Could you check a few things on this model? Use its own coordinates, in mm. A direction names the side the tool comes from. Give positions to 0.01 mm unless a question says otherwise; leave off trailing zeros. Loops run counter-clockwise (first coordinate to the right, second up) from the corner with the lowest first, then second, coordinate; pieces in that order, holes last. Notation, with made-up numbers: (44.5, 33) - (89.5, 33) arc R32 ccw to (89.5, 72) - close; hole circle Ø9 at (36, 44). An arc over 180 degrees is marked (long way). Use CSV: the item, a comma, the result in double quotes.
from build123d import *

# Parameters (mm, degrees)
BOSS_EXTRUDE1_DEPTH      = 30
BOSS_EXTRUDE1_DEPTH_BACK = 30
BOSS_EXTRUDE2_DEPTH      = 3.2
SKETCH3_R                = 1.35
CUT_EXTRUDE1_DEPTH       = 86.695011246
SKETCH4_R                = 6.35
SKETCH4_R_2              = 1.35
BOSS_EXTRUDE3_DEPTH      = 6
CHAMFER1_SIZE            = 6
FILLET1_R                = 5
SKETCH5_W                = 2.4
SKETCH5_H                = 8
BOSS_EXTRUDE4_DEPTH      = 60
FILLET2_R                = 5
FILLET3_R                = 10


with BuildPart() as part:
    # Sketch1 → Boss-Extrude1 (new, two sides: drawn at the far end of the back side and taken through both)
    with BuildSketch(Plane(origin=(0, 0, 0), x_dir=(0, 0, -1), z_dir=(1, 0, 0)).offset(-BOSS_EXTRUDE1_DEPTH_BACK)):
        Polygon((-8, 54.174772512), (-46.414198462, 60.948232143), (-46.414198462, 57.901952308), (-1.6, 50), (-1.6, 0), (0, 0), (0, 50), align=None)
    extrude(amount=BOSS_EXTRUDE1_DEPTH + BOSS_EXTRUDE1_DEPTH_BACK)

    # Sketch2 → Boss-Extrude2 (add)
    with BuildSketch(Plane(origin=(30, 0, 0), x_dir=(0, 0, -1), z_dir=(1, 0, 0))):
        Polygon((0, 0), (0, 107.45890736), (-46.414198462, 107.45890736), (-46.414198462, 57.901952308), (-1.6, 0), align=None)
    boss_extrude2 = extrude(amount=BOSS_EXTRUDE2_DEPTH)

    # Mirror1: Boss-Extrude2 across plane
    add(boss_extrude2.mirror(Plane(origin=(0, 0, 0), x_dir=(0, 0, 1), z_dir=(1, 0, 0))))

    # Sketch3 → Cut-Extrude1 (cut, through all)
    with BuildSketch(Plane(origin=(0, 51.173122664, -9.023202213), x_dir=(1, 0, 0), z_dir=(0, 0.984807753012208, -0.17364817766693144))):
        with Locations(Location((0, -45.21547888, 0), (0, 0, 270))):
            Circle(SKETCH3_R)
    extrude(amount=-CUT_EXTRUDE1_DEPTH, mode=Mode.SUBTRACT)

    # Sketch4 → Boss-Extrude3 (add)
    with BuildSketch(Plane(origin=(0, 48.218699405, -8.50225768), x_dir=(1, 0, 0), z_dir=(0, -0.9848077530122079, 0.1736481776669319))):
        with Locations(Location((0, 45.21547888, 0), (0, 0, 90))):
            Circle(SKETCH4_R)
        with Locations(Location((0, 45.21547888, 0), (0, 0, 90))):
            Circle(SKETCH4_R_2, mode=Mode.SUBTRACT)
    extrude(amount=BOSS_EXTRUDE3_DEPTH)

    # Chamfer1
    # the kernel refuses this chamfer: 6 mm, written as the material it adds along each edge
    with BuildSketch(Plane(origin=(0, 56.070284915, 36.026296477), x_dir=(0, 0.1736481776669323, 0.9848077530122077), z_dir=(1, 0, 0))) as chamfer1_piece_1_section:
        Polygon((6.35 + CHAMFER1_SIZE, 0), (6.35, CHAMFER1_SIZE), (6.35, 0), align=None)
    chamfer1_piece_1 = revolve(axis=Axis((0, 56.070284915, 36.026296477), (0, -0.9848077530122079, 0.1736481776669319)), mode=Mode.PRIVATE)
    chamfer1_piece_1 = split(chamfer1_piece_1, bisect_by=Plane(origin=(0, 51.643480969, 46.414198462), z_dir=(0, 0, -1)), keep=Keep.TOP, mode=Mode.PRIVATE)
    chamfer1_piece_1 = split(chamfer1_piece_1, bisect_by=Plane(origin=(0, 48.535444939, 27.846718406), z_dir=(0, 0.9848077530122079, -0.1736481776669319)), keep=Keep.TOP, mode=Mode.PRIVATE)
    add(chamfer1_piece_1)

    # Fillet1
    fillet1_edges = [part.edges().sort_by_distance(p)[0] for p in [
        (0, 50, 1.6),
        (-30, 53.950976154, 24.007099231),
        (30, 53.950976154, 24.007099231),
        (-30, 25, 1.6),
        (30, 25, 1.6),
    ]]
    fillet(fillet1_edges, radius=FILLET1_R)

    # Sketch5 → Boss-Extrude4 (add)
    with BuildSketch(Plane.ZY.offset(-30)):
        with Locations((1.2, 103.45890736)):
            Rectangle(SKETCH5_W, SKETCH5_H)
    extrude(amount=BOSS_EXTRUDE4_DEPTH)

    # Fillet2
    fillet2_edges = [part.edges().sort_by_distance(p)[0] for p in [
        (30, 103.45890736, 2.4),
        (-30, 103.45890736, 2.4),
    ]]
    fillet(fillet2_edges, radius=FILLET2_R)

    # Fillet3
    fillet3_edges = [part.edges().sort_by_distance(p)[0] for p in [
        (31.6, 107.45890736, 46.414198462),
        (-31.6, 107.45890736, 46.414198462),
    ]]
    fillet(fillet3_edges, radius=FILLET3_R)


solid = part.part
1) I'm going to push flat-ended pins straight in: P1, Ø8, axis at x = -22.5, z = 34.5, coming from the -Y side; P2, Ø6, axis at x = -2, z = 19, coming from the +Y side; P3, Ø1.5, axis at x = 2.5, z = 5.5, coming from the -Y side. Where does each tip first touch, or does it pass through?
Answer below:
P1,"stops at y = 55.1"
P2,"stops at y = 56.64"
P3,"stops at y = 50.45"
2) Which directions (+Z, -Z, +X, -X, +Y, -Y) give clear straight access to the entire face, cutting with the end or side of a thin tool? Please do faces 5 (the cylindrical face through (0.35, 49.056, 2.801)), 6 (the flat face through (-2, 107.459, 2)), 7 (the flat face through (0, 103, 2.4)), 8 (the flat face through (-30, 35, 17)).
Answer below:
face 5,"-Y"
face 6,"+Z, -Z, +X, -X, +Y"
face 7,"+Z, +Y"
face 8,"+Z, -Y"
3) We'd pull the mould along Y, two halves only. Please class faces 1 (the flat face through (-0.42, 52.058, 3.944)), 2 (the cylindrical face through (28.5, 52.86, 26.04)), 3 (the flat face through (0, 60, 46.414)), 4 (the flat face through (0, 99.459, 1)): +Y half, -Y half, draft (parallel to the pull), parting line (faces both ways), or undercut.
Answer below:
face 1,"undercut"
face 2,"-Y half"
face 3,"draft"
face 4,"undercut"
4) Suppose I cut it at A-A (x = 18.5). Please give me the cut outline in (y, z), plus the area to 3 significant figures.
Answer below:
outline,"(0, 0) - (50, 0) - (54.17, 8) - (60.95, 46.41) - (57.9, 46.41) - (50.73, 5.73) arc R5 cw to (45.8, 1.6) - (0, 1.6) - close; (99.46, 0) - (107.46, 0) - (107.46, 2.4) - (99.46, 2.4) - close"
area,"233 mm2"
5) Suppose I cut it at C-C (y = 35.5). Please give me the cut outline in (x, z).
Answer below:
outline,"(-33.2, 0) - (33.2, 0) - (33.2, 29.08) - (30, 29.08) - (30, 6.6) arc R5 cw to (25, 1.6) - (-25, 1.6) arc R5 cw to (-30, 6.6) - (-30, 29.08) - (-33.2, 29.08) - close"
6) I need wall thicknesses on line 1 along X through (y, z) = (63, 32.5); line 2 along Z through (x, y) = (16, 24); line 3 along X through (y, z) = (23.5, 5). Which ranges of each line are inside material? Lowest first, please.
Answer below:
line 1,"x = -33.2 to -30, 30 to 33.2"
line 2,"z = 0 to 1.6"
line 3,"x = -33.2 to -29.74, 29.74 to 33.2"
7) Suppose I cut it at D-D (x = -27). Please give me the cut outline in (y, z).
Answer below:
outline,"(0, 0) - (50, 0) - (54.17, 8) - (60.95, 46.41) - (57.9, 46.41) - (57.41, 46.03) - (50.32, 5.8) arc R4.58 cw to (45.8, 2.02) - (0.54, 2.02) - (0, 1.6) - close; (99.46, 0) - (107.46, 0) - (107.46, 2.82) - (99.46, 2.82) - close"
8) Suppose I cut it at B-B (y = 63.5). Please give me the cut outline in (x, z), plus the area to 3 significant figures.
Answer below:
outline,"(-33.2, 0) - (-30, 0) - (-30, 46.41) - (-33.2, 46.41) - close; (30, 0) - (33.2, 0) - (33.2, 46.41) - (30, 46.41) - close"
area,"297 mm2"
